For this review, take the finished solid that the model builds, in its own axes (mm). A direction names the side the tool comes from. Coordinates: 2 decimals unless noted, no trailing zeros. Write each loop counter-clockwise with the first axis right and the second up, starting at its lowest first coordinate (ties: lowest second). Pieces come first, ordered by that corner, then holes. Notation, with made-up numbers: M -3,39.5 L 2,39.5 A27 cw 2,66.5 Z; hole C 83.25,1.5 d6. An arc over 180 degrees is marked long. One line per question, with ' | ' between items.
from build123d import *

# Parameters (mm, degrees)
SKETCH1_R           = 40
SKETCH1_R_2         = 8.5
BOSS_EXTRUDE1_DEPTH = 2.5
FILLET2_R           = 2
CIRPATTERN1_COUNT   = 5
SKETCH6_R           = 13
SKETCH6_R_2         = 8.5
BOSS_EXTRUDE2_DEPTH = 5


with BuildPart() as part:
    # Sketch1 → Boss-Extrude1 (new body, symmetric)
    with BuildSketch(Plane.XY):
        Circle(SKETCH1_R)
        Circle(SKETCH1_R_2, mode=Mode.SUBTRACT)
    extrude(amount=BOSS_EXTRUDE1_DEPTH, both=True)

    # Fillet2
    fillet2_edges = [part.edges().sort_by_distance(p)[0] for p in [
        (-40, 0, 2.5),
    ]]
    fillet(fillet2_edges, radius=FILLET2_R)

    # Sketch5 → CSK for M2 Flat Head Machine Screw1 (revolve, cut)
    with BuildSketch(Plane(origin=(-2.162785463, 32.427956443, 2.5), x_dir=(0, -1, 0), z_dir=(1, 0, 0))):
        Polygon((0, 0), (0, 5), (1.225, 5), (1.2, 4.975), (1.2, 2), (3.2, 0), align=None)
    csk_for_m2_flat_head_machine_screw1 = revolve(axis=Axis((-2.162785463, 32.427956443, 8.85), (0, 0, -1)), mode=Mode.SUBTRACT)

    # CirPattern1: CSK for M2 Flat Head Machine Screw1 ×5 about axis
    cirpattern1_axis = Axis((0, 0, 0), (0, 0, 1))
    for i in range(1, CIRPATTERN1_COUNT):
        add(csk_for_m2_flat_head_machine_screw1.rotate(cirpattern1_axis, i * 360 / CIRPATTERN1_COUNT), mode=Mode.SUBTRACT)

    # Sketch6 → Boss-Extrude2 (add)
    with BuildSketch(Plane.XY.offset(2.5)):
        Circle(SKETCH6_R)
        Circle(SKETCH6_R_2, mode=Mode.SUBTRACT)
    extrude(amount=BOSS_EXTRUDE2_DEPTH)


solid = part.part
1) To check wall thickness, follow line 1 along Y through (x, z) = (0, 6); line 2 along Z through (x, y) = (22.5, 13); line 3 along X through (y, z) = (33, 1.25). State the ranges of each line that lie inside material, in increasing order. Write a range as [from, to].
Responses:
line 1: [-13, -8.5], [8.5, 13] | line 2: [-2.5, 2.5] | line 3: [-22.35, -4.03], [-0.3, 22.35]
2) Machinability: for faces 1 (the cylindrical face through (4.57, 7.167, 2.43)), 2 (the flat face through (16, 1, 2.5)), which of the approach directions +Z, -Z, +X, -X, +Y, -Y give a long, thin tool a straight path to every point of the face, cutting with its end or side? Answer none if there is none.
Responses:
face 1: +Z, -Z | face 2: +Z
3) The part is to be moulded in two halves that separate along Y. For faces 3 (the cylindrical face through (-10.316, -7.91, 4.965)), 4 (the flat face through (-1, 9, -2.5)), 5 (the cylindrical face through (-16.113, -27.579, -0.967)), say which applies: +Y half, -Y half, draft (parallel to the pull), parting line (faces both ways), or undercut.
Responses:
face 3: parting line | face 4: draft | face 5: undercut
4) Insertion check: pin 1 Ø4 at (x, y) = (16, 20.5) entering from +Z; pin 2 Ø6 at (y, z) = (14.5, 1.5) entering from +X; pin 3 Ø6 at (y, z) = (19.5, -0.5) entering from -X. Each pin has a flat end and moves straight along its axis. Give the tip position at first contact, or say it passes through.
Responses:
pin 1: z = 2.5 | pin 2: x = 38.27 | pin 3: x = -36.44
5) We need section A-A on y = 0. State the section outline as (x, z) points, then the cut area to 3 significant figures.
Responses:
outline: M -40,-2.5 L -8.5,-2.5 L -8.5,7.5 L -13,7.5 L -13,2.5 L -38,2.5 A2 ccw -40,0.5 Z; M 8.5,-2.5 L 40,-2.5 L 40,0.5 A2 ccw 38,2.5 L 13,2.5 L 13,7.5 L 8.5,7.5 Z | area: 358 mm^2
6) We need section B-B on z = -1. State the section outline as (x, y) points, then the cut area to 3 significant figures.
Responses:
outline: C 0,0 d80; hole C -31.51,7.96 d2.4; hole C -17.31,-27.51 d2.4; hole C 0,0 d17; hole C -2.16,32.43 d2.4; hole C 20.81,-24.96 d2.4; hole C 30.17,12.08 d2.4 | area: 4,780 mm^2
